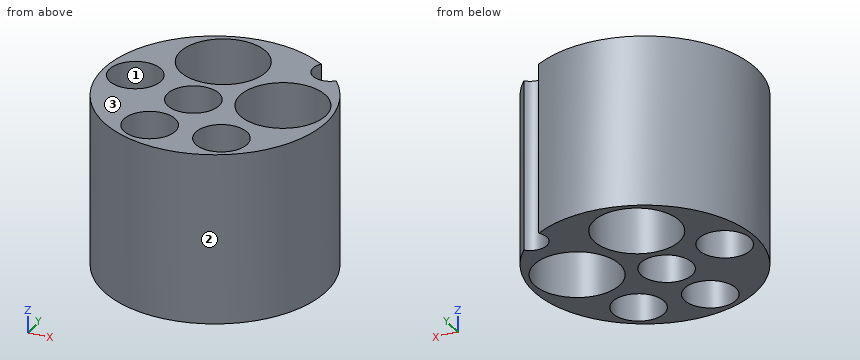
```python
from build123d import *

# Parameters (mm, degrees)
F0_R     = 6.5
F1_DEPTH = 10
F3_R     = 2.5
F3_R_2   = 1.5
F3_R_3   = 1
F4_DEPTH = 25
F5_DEPTH = 15


with BuildPart() as f1:
    # F0 (on Top) → F1 (new body)
    with BuildSketch(Plane.XY):
        Circle(F0_R)
    extrude(amount=F1_DEPTH)

    # F3 (on offset) → F4 (cut, symmetric)
    with BuildSketch(Plane.XY.offset(10)):
        with Locations((-1.288395, 3.468435)):
            Circle(F3_R)
        with Locations((-4.699119, 0.091015)):
            Circle(F3_R_2)
        with Locations((-0.794072, -0.917286)):
            Circle(F3_R_2)
        with Locations((4.178119, 4.979289)):
            Circle(F3_R_3)
        with Locations((3.64795, 0.618435)):
            Circle(F3_R)
        with Locations((2.428381, -4.024049)):
            Circle(F3_R_2)
        with Locations((-1.550249, -4.436973)):
            Circle(F3_R_2)
    extrude(amount=F4_DEPTH, both=True, mode=Mode.SUBTRACT)

    # F3 (on offset) → F5 (cut, symmetric)
    with BuildSketch(Plane.XY.offset(10)):
        with Locations((4.178119, 4.979289)):
            Circle(F3_R_3)
    extrude(amount=F5_DEPTH, both=True, mode=Mode.SUBTRACT)


solid = f1.part
```
Read the model definition and answer for the solid it produces. Units are mm, in the model's axes. Face numbers are marked on the shaded views. Give positions to 0.01 mm unless a question says otherwise; leave off trailing zeros. Write each loop counter-clockwise with the first axis right and the second up, starting at its lowest first coordinate (ties: lowest second). Pieces come first, ordered by that corner, then holes. Notation, with made-up numbers: (20, 54) - (60, 54) arc R15 ccw to (60, 64) - close; hole circle Ø7 at (78.5, 31). An arc over 180 degrees is marked (long way). Write item = value, one per line. Start each with the question number.
Item 1: The mould has two halves that part along Y. Classify the marked faces 1, 2 and 3: +Y half, -Y half, draft (parallel to the pull), parting line (faces both ways), or undercut.
Item 2: Find section C-C (x = -5). Give the vertices of the cut face in (y, z), then the cut area to 3 significant figures.
Item 3: Find section D-D (y = 2). Give the vertices of the cut face in (x, z).
Item 4: Each of these flat-tipped pins is pushed along its axis until it touches: P1, Ø1, axis at x = 4, z = 5.5, coming from the -Y side; P2, Ø1, axis at x = -2, z = 4.5, coming from the +Y side. Where does it stop, or does it pass through?
Item 5: Find section B-B (z = 5). Give the vertices of the cut face in (x, y).
Item 6: Find the intervals of material crossed by probe 1 along Y at (x, z) = (-0.25, 3.75); probe 2 along X at (y, z) = (-4, 6.25); probe 3 along X at (y, z) = (1.75, 1.5), in increasing order. Write a range as [from, to].
Item 7: Find section A-A (x = -0.5). Give the vertices of the cut face in (y, z).
Response:
q1.face_1 = undercut
q1.face_2 = parting line
q1.face_3 = draft
q2.outline = (-4.15, 0) - (-1.38, 0) - (-1.38, 10) - (-4.15, 10) - close; (1.56, 0) - (4.15, 0) - (4.15, 10) - (1.56, 10) - close
q2.area = 53.7 mm²
q3.outline = (-6.18, 0) - (-3.31, 0) - (-3.31, 10) - (-6.18, 10) - close; (0.73, 0) - (1.56, 0) - (1.56, 10) - (0.73, 10) - close; (5.73, 0) - (6.18, 0) - (6.18, 10) - (5.73, 10) - close
q4.P1 = -5.48
q4.P2 = 6.32
q5.outline = (3.36, 5.56) arc R6.5 ccw (long way) to (4.89, 4.28) arc R1 cw to start; hole circle Ø3 at (-4.7, 0.09); hole circle Ø5 at (-1.29, 3.47); hole circle Ø3 at (-1.55, -4.44); hole circle Ø3 at (-0.79, -0.92); hole circle Ø3 at (2.43, -4.02); hole circle Ø5 at (3.65, 0.62)
q6.probe_1 = [-6.5, -5.18], [-3.69, -2.32], [0.48, 1.19], [5.74, 6.5]
q6.probe_2 = [-5.12, -2.99], [-0.12, 0.93], [3.93, 5.12]
q6.probe_3 = [-6.26, -3.1], [0.53, 1.42], [5.88, 6.26]
q7.outline = (-6.48, 0) - (-5.51, 0) - (-5.51, 10) - (-6.48, 10) - close; (-3.37, 0) - (-2.39, 0) - (-2.39, 10) - (-3.37, 10) - close; (0.55, 0) - (1.1, 0) - (1.1, 10) - (0.55, 10) - close; (5.84, 0) - (6.48, 0) - (6.48, 10) - (5.84, 10) - close
